from build123d import *

# Parameters (mm, degrees)
SKETCH_1_W          = 45
SKETCH_1_H          = 35
EXTRUDE_1_DEPTH     = 7
SKETCH_2_R          = 2
CUT_EXTRUDE_1_DEPTH = 7
FILLET_1_R          = 2
SKETCH_3_R          = 1.5
EXTRUDE_2_DEPTH     = 8
SKETCH_3_2_R        = 1.5
CUT_EXTRUDE_2_DEPTH = 3


with BuildPart() as part:
    # Sketch 1 → Extrude 1 (new body)
    with BuildSketch(Plane(origin=(0, 0, 0), x_dir=(1, 0, 0), z_dir=(0, 1, 0))):
        Rectangle(SKETCH_1_W, SKETCH_1_H)
    extrude(amount=EXTRUDE_1_DEPTH)

    # Sketch 2 → Cut-Extrude 1 (cut)
    with BuildSketch(Plane(origin=(0, 7, 0), x_dir=(1, 0, 0), z_dir=(0, 1, 0))):
        with Locations(Location((20.3, 15.3, 0), (0, 0, 270))):
            Circle(SKETCH_2_R)
        with Locations(Location((20.3, -15.3, 0), (0, 0, 270))):
            Circle(SKETCH_2_R)
    extrude(amount=-CUT_EXTRUDE_1_DEPTH, mode=Mode.SUBTRACT)

    # Fillet 1
    fillet_1_edges = [part.edges().sort_by_distance(p)[0] for p in [
        (22.5, 3.5, 17.5),
        (-22.5, 3.5, 17.5),
        (-22.5, 3.5, -17.5),
        (22.5, 3.5, -17.5),
    ]]
    fillet(fillet_1_edges, radius=FILLET_1_R)

    # Sketch 3 → Extrude 2 (add, symmetric)
    with BuildSketch(Plane(origin=(0, 0, 0), x_dir=(0, 0, -1), z_dir=(1, 0, 0))):
        with BuildLine():
            Line((0.005, 7), (-4.995, 7))
            Line((-4.995, 7), (-4.995, 17))
            ThreePointArc((-4.995, 17), (0.005, 22), (5.005, 17))
            Line((5.005, 17), (5.005, 7))
            Line((5.005, 7), (0.005, 7))
        make_face()
        with Locations((0.005, 17)):
            Circle(SKETCH_3_R, mode=Mode.SUBTRACT)
    extrude(amount=EXTRUDE_2_DEPTH, both=True)

    # Sketch 3_2 → Cut-Extrude 2 (cut, symmetric)
    with BuildSketch(Plane(origin=(0, 0, 0), x_dir=(0, 0, -1), z_dir=(1, 0, 0))):
        with BuildLine():
            Line((0.005, 7), (-4.995, 7))
            Line((-4.995, 7), (-4.995, 17))
            ThreePointArc((-4.995, 17), (0.005, 22), (5.005, 17))
            Line((5.005, 17), (5.005, 7))
            Line((5.005, 7), (0.005, 7))
        make_face()
        with Locations((0.005, 17)):
            Circle(SKETCH_3_2_R, mode=Mode.SUBTRACT)
    extrude(amount=CUT_EXTRUDE_2_DEPTH, both=True, mode=Mode.SUBTRACT)


solid = part.part
For this review, take the finished solid that the model builds, in its own axes (mm). A direction names the side the tool comes from. Coordinates: 2 decimals unless noted, no trailing zeros. Order: outer loops, then holes, each group sorted by start corner. A loop starts at its lowest first (then second) coordinate and runs counter-clockwise, first axis right, second up. Notation, with made-up numbers: (26.25, 49) - (76.25, 49) arc R8 ccw to (76.25, 58) - close; hole circle Ø2 at (24.5, 28.25). An arc over 180 degrees is marked (long way). Use one line per item in the form item = value.
Q1. For faces 1 (the flat face through (-8, 15, 0)), 2 (the flat face through (8, 15, 0)), 3 (the flat face through (-5, 12, 4.995)), list the 3-axis set-ups (+Z, -Z, +X, -X, +Y, -Y) from which the entire face can be reached by the end or side of a thin tool; tool diameter is ignored.
Checked values:
face_1 = +Z, -Z, -X, +Y
face_2 = +Z, -Z, +X, +Y
face_3 = +Z, +X, -X, +Y
Q2. For probe 1 along X at (y, z) = (3.25, -15.3); probe 2 along X at (y, z) = (9.25, -2); probe 3 along Y at (x, z) = (8, 9.5), list the stretches that pass through material, from the lowest coordinate up. Write a range as from..to.
Checked values:
probe_1 = -22.5..18.3, 22.3..22.5
probe_2 = -8..-3, 3..8
probe_3 = 0..7
Q3. For P1, Ø2.5, axis at y = 17, z = -0.005, coming from the -X side; P2, Ø6.5, axis at x = 20.3, z = -15.3, coming from the +Y side; P3, Ø8, axis at y = 12, z = 1, coming from the +X side; P4, Ø2.5, axis at x = -6, y = 11.5, coming from the -Z side (3 decimals), all flat-tipped, find the tip position at first contact; note any pin that passes through.
Checked values:
P1 = through
P2 = 7
P3 = 8
P4 = -5.005
Q4. Consider section C-C (x = 5). Give the boundary of the cut face in (y, z) (3 decimals), then the cut area to 3 significant figures.
Checked values:
outline = (0, -17.5) - (7, -17.5) - (7, -5.005) - (17, -5.005) arc R5 ccw to (17, 4.995) - (7, 4.995) - (7, 17.5) - (0, 17.5) - close; hole circle Ø3 at (17, -0.005)
area = 377 mm2
Q5. Consider section A-A (y = 3). Give the boundary of the cut face in (x, z), then the cut area to 3 significant figures.
Checked values:
outline = (-22.5, -15.5) arc R2 ccw to (-20.5, -17.5) - (20.5, -17.5) arc R2 ccw to (22.5, -15.5) - (22.5, 15.5) arc R2 ccw to (20.5, 17.5) - (-20.5, 17.5) arc R2 ccw to (-22.5, 15.5) - close; hole circle Ø4 at (20.3, -15.3); hole circle Ø4 at (20.3, 15.3)
area = 1,550 mm2
Q6. Consider section D-D (x = -18.5). Give the boundary of the cut face in (y, z), then the cut area to 3 significant figures.
Checked values:
outline = (0, -17.5) - (7, -17.5) - (7, 17.5) - (0, 17.5) - close
area = 245 mm2
Q7. Draft analysis for pull direction Z (two halves, no side actions). For faces 4 (the cylindrical face through (-21.93, 3.55, -16.9)), 5 (the cylindrical face through (20.388, 3.549, 13.302)), 6 (the flat face through (3, 15, 0)), state which applies: +Z half, -Z half, draft (parallel to the pull), parting line (faces both ways), or undercut.
Checked values:
face_4 = -Z half
face_5 = undercut
face_6 = draft
Q8. Consider section B-B (y = 11.75). Give the boundary of the cut face in (x, z) (3 decimals).
Checked values:
outline = (-8, -5.005) - (-3, -5.005) - (-3, 4.995) - (-8, 4.995) - close; (3, -5.005) - (8, -5.005) - (8, 4.995) - (3, 4.995) - close
